Build history of the part. All positions in model axes, mm. A direction names the side the tool comes from. Round coordinates to 2 decimals unless told otherwise and drop trailing zeros. Order: outer loops, then holes, each group sorted by start corner. A loop starts at its lowest first (then second) coordinate and runs counter-clockwise, first axis right, second up. Notation, with made-up numbers: (28, 56) -> (69, 56) arc R26 cw to (69, 84) -> close; hole circle Ø4 at (-24.75, 8.5). An arc over 180 degrees is marked (long way). Answer as a JSON object with one key per item and string values.
from build123d import *

# Parameters (mm, degrees)
CROQUIS1_R               = 2
CROQUIS1_R_2             = 1.5
CROQUIS1_W               = 75
CROQUIS1_H               = 50
SALIENTE_EXTRUIR4_DEPTH  = 5
CROQUIS3_W               = 5
CROQUIS3_H               = 5
SALIENTE_EXTRUIR5_DEPTH  = 50
CROQUIS4_W               = 3
CROQUIS4_H               = 50
SALIENTE_EXTRUIR7_DEPTH  = 22
SALIENTE_EXTRUIR9_DEPTH  = 27.5
CROQUIS7_W               = 10
CROQUIS7_H               = 5
SALIENTE_EXTRUIR10_DEPTH = 10
CROQUIS8_W               = 10
CROQUIS8_H               = 5
SALIENTE_EXTRUIR11_DEPTH = 10


with BuildPart() as part:
    # Croquis1 → Saliente-Extruir4 (new body)
    # profile 1 of 2: a face of its own
    with BuildSketch(Plane.XY):
        Polygon((-71.5, -27.5), (-71.5, -32.5), (-3.5, -32.5), (-3.5, -27.5), (1.5, -27.5), (1.5, -25), (1.5, 25), (1.5, 27.5), (-3.5, 27.5), (-3.5, 32.5), (-71.5, 32.5), (-71.5, 27.5), (-76.5, 27.5), (-76.5, -27.5), align=None)
        with Locations((-66.5, -22.5)):
            Circle(CROQUIS1_R, mode=Mode.SUBTRACT)
        with Locations((-2, 0)):
            Circle(CROQUIS1_R_2, mode=Mode.SUBTRACT)
        with Locations((-66.5, 22.5)):
            Circle(CROQUIS1_R, mode=Mode.SUBTRACT)
    # profile 2 of 2: a face of its own
    with BuildSketch(Plane.XY):
        with Locations((39, 0)):
            Rectangle(CROQUIS1_W, CROQUIS1_H)
    extrude(amount=SALIENTE_EXTRUIR4_DEPTH)

    # Croquis3 → Saliente-Extruir5 (add)
    with BuildSketch(Plane(origin=(0, 0, 0), x_dir=(-1, 0, 0), z_dir=(0, 0, -1))):
        with Locations((74, 30)):
            Rectangle(CROQUIS3_W, CROQUIS3_H)
        with Locations((1, -30)):
            Rectangle(CROQUIS3_W, CROQUIS3_H)
        with Locations((1, 30)):
            Rectangle(CROQUIS3_W, CROQUIS3_H)
        with Locations((74, -30)):
            Rectangle(CROQUIS3_W, CROQUIS3_H)
    extrude(amount=-SALIENTE_EXTRUIR5_DEPTH)

    # Croquis4 → Saliente-Extruir7 (add)
    with BuildSketch(Plane.XY.offset(5)):
        with Locations((56, 0)):
            Rectangle(CROQUIS4_W, CROQUIS4_H)
    extrude(amount=SALIENTE_EXTRUIR7_DEPTH)

    # Croquis6 → Saliente-Extruir9 (add)
    with BuildSketch(Plane(origin=(0, 0, 0), x_dir=(-1, 0, 0), z_dir=(0, 0, -1))):
        Polygon((-31.5, 13.5), (-31.5, 14.5), (-41.5, 14.5), (-41.5, 13.5), (-41.5, 9.5), (-31.5, 9.5), align=None)
        Polygon((-31.5, -13.5), (-31.5, -9.5), (-41.5, -9.5), (-41.5, -13.5), (-41.5, -14.5), (-31.5, -14.5), align=None)
    extrude(amount=SALIENTE_EXTRUIR9_DEPTH)

    # Croquis7 → Saliente-Extruir10 (add)
    with BuildSketch(Plane(origin=(0, 14.5, 0), x_dir=(1, 0, 0), z_dir=(0, 1, 0))):
        with Locations((36.5, 25)):
            Rectangle(CROQUIS7_W, CROQUIS7_H)
    extrude(amount=SALIENTE_EXTRUIR10_DEPTH)

    # Croquis8 → Saliente-Extruir11 (add)
    with BuildSketch(Plane.XZ.offset(14.5)):
        with Locations((36.5, -25)):
            Rectangle(CROQUIS8_W, CROQUIS8_H)
    extrude(amount=SALIENTE_EXTRUIR11_DEPTH)


solid = part.part
1) Flat gauge pins, fed straight in: pin 1 Ø11 at (x, z) = (36.5, -11) entering from -Y; pin 2 Ø8 at (x, y) = (35.5, -18) entering from +Z; pin 3 Ø4.5 at (y, z) = (-17, -13.5) entering from -X; pin 4 Ø4 at (y, z) = (9.5, 21) entering from -X. Where does each tip first touch, or does it go through?
Checked values:
{"pin 1": "stops at y = -14.5", "pin 2": "stops at z = 5", "pin 3": "passes through", "pin 4": "stops at x = 54.5"}
2) Cut at B-B, the plane x = -2. Give the cut face in (y, z), plus the area to 3 significant figures.
Checked values:
{"outline": "(-32.5, 0) -> (-1.5, 0) -> (-1.5, 5) -> (-27.5, 5) -> (-27.5, 50) -> (-32.5, 50) -> close; (1.5, 0) -> (32.5, 0) -> (32.5, 50) -> (27.5, 50) -> (27.5, 5) -> (1.5, 5) -> close", "area": "760 mm²"}
3) Cut at C-C, the plane z = 21.5. Give the cut face in (x, y).
Checked values:
{"outline": "(-76.5, -32.5) -> (-71.5, -32.5) -> (-71.5, -27.5) -> (-76.5, -27.5) -> close; (-76.5, 27.5) -> (-71.5, 27.5) -> (-71.5, 32.5) -> (-76.5, 32.5) -> close; (-3.5, -32.5) -> (1.5, -32.5) -> (1.5, -27.5) -> (-3.5, -27.5) -> close; (-3.5, 27.5) -> (1.5, 27.5) -> (1.5, 32.5) -> (-3.5, 32.5) -> close; (54.5, -25) -> (57.5, -25) -> (57.5, 25) -> (54.5, 25) -> close"}
4) Probe L1, parallel to Y at x = -2, z = 2.9; L2, parallel to Y at x = 37, z = -19.5; L3, parallel to X at y = 18, z = 6. List the from-to ranges inside material, lowest first. Write a range as from..to.
Checked values:
{"L1": "y = -32.5..-1.5, 1.5..32.5", "L2": "y = -14.5..-9.5, 9.5..14.5", "L3": "x = 54.5..57.5"}
5) Which spindle directions (+Z, -Z, +X, -X, +Y, -Y) get a long thin tool onto all of the face, cutting with end or side? Do faces 5 (the face through (36, 14.5, -11)), 6 (the face through (42, -25, 4)), 7 (the face through (-1, -27.5, 27)), 8 (the face through (-3.5, 30, 27)). Say none if no direction does.
Checked values:
{"face 5": "+X, -X, +Y", "face 6": "+Z, -Z, +X, -Y", "face 7": "+Z, +X, -X", "face 8": "+Z, +Y, -Y"}
6) Cut at A-A, the plane y = 0. Give the cut face in (x, z), plus the area to 3 significant figures.
Checked values:
{"outline": "(-76.5, 0) -> (-3.5, 0) -> (-3.5, 5) -> (-76.5, 5) -> close; (-0.5, 0) -> (76.5, 0) -> (76.5, 5) -> (57.5, 5) -> (57.5, 27) -> (54.5, 27) -> (54.5, 5) -> (-0.5, 5) -> close", "area": "816 mm²"}
7) Cut at D-D, the plane y = -22.5. Give the cut face in (x, z), plus the area to 3 significant figures.
Checked values:
{"outline": "(-76.5, 0) -> (-68.5, 0) -> (-68.5, 5) -> (-76.5, 5) -> close; (-64.5, 0) -> (76.5, 0) -> (76.5, 5) -> (57.5, 5) -> (57.5, 27) -> (54.5, 27) -> (54.5, 5) -> (-64.5, 5) -> close; (31.5, -27.5) -> (41.5, -27.5) -> (41.5, -22.5) -> (31.5, -22.5) -> close", "area": "861 mm²"}
8) Pull direction Z, two halves, no side cores. Call faces 1 (the face through (36, -19, -22.5)), 2 (the face through (67, 0, 5)), 3 (the face through (36, -17, -27.5)), 4 (the face through (-66.76, -20.517, 2.465)): pulls with the +Z half, pulls with the -Z half, needs draft (parallel to the pull), parting line crosses it, or undercut.
Checked values:
{"face 1": "undercut", "face 2": "pulls with the +Z half", "face 3": "pulls with the -Z half", "face 4": "needs draft"}
